Source: CAD feature listing. Evaluate the final solid. Frame: model axes, mm. A direction names the side the tool comes from. Give positions to 0.01 mm unless a question says otherwise; leave off trailing zeros. Loops run counter-clockwise (first coordinate to the right, second up) from the corner with the lowest first, then second, coordinate; pieces in that order, holes last.
```python
from build123d import *

# Parameters (mm, degrees)
RESSALTO_EXTRUS_O1_DEPTH = 3
ESBO_O2_W                = 40
ESBO_O2_H                = 3
ESBO_O2_W_2              = 3
ESBO_O2_H_2              = 40
CORTE_EXTRUS_O1_DEPTH    = 436.556992799
ESBO_O3_R                = 1.5
CORTE_EXTRUS_O2_DEPTH    = 436.556992799


with BuildPart() as part:
    # Esboço1 → Ressalto-extrusão1 (new body)
    with BuildSketch(Plane.XY):
        with BuildLine():
            Line((-241.20368795, -59.651351358), (-241.20368795, -29.651351358))
            ThreePointArc((-241.20368795, -29.651351358), (-246.107895674, -13.213553147), (-259.217101951, -2.150046733))
            ThreePointArc((-259.217101951, -2.150046733), (-264.561513741, -3.018769002), (-265.981323334, -8.243858139))
            ThreePointArc((-265.981323334, -8.243858139), (-265.003447457, -13.909864328), (-265.583076332, -19.630344878))
            ThreePointArc((-265.583076332, -19.630344878), (-271.11591561, -26.364097317), (-279.829636843, -26.200406546))
            ThreePointArc((-279.829636843, -26.200406546), (-306.442768457, 34.527322411), (-252.007526665, 72.381256019))
            ThreePointArc((-252.007526665, 72.381256019), (-244.422773084, 74.999120757), (-241.20368795, 82.348895826))
            Line((-241.20368795, 82.348895826), (-241.20368795, 98.348401458))
            ThreePointArc((-241.20368795, 98.348401458), (-237.984602816, 105.698176528), (-230.399849235, 108.316041265))
            ThreePointArc((-230.399849235, 108.316041265), (-175.964607443, 146.169974874), (-202.577739058, 206.897703831))
            ThreePointArc((-202.577739058, 206.897703831), (-211.29146029, 207.061394601), (-216.824299569, 200.327642163))
            ThreePointArc((-216.824299569, 200.327642163), (-217.403928444, 194.607161612), (-216.426052566, 188.941155423))
            ThreePointArc((-216.426052566, 188.941155423), (-217.845862159, 183.716066286), (-223.190273949, 182.847344017))
            ThreePointArc((-223.190273949, 182.847344017), (-236.299480227, 193.910850432), (-241.20368795, 210.348648642))
            Line((-241.20368795, 210.348648642), (-241.20368795, 240.348648642))
            Line((-241.20368795, 240.348648642), (-211.20368795, 240.348648642))
            ThreePointArc((-211.20368795, 240.348648642), (-194.76588974, 245.252856366), (-183.702383325, 258.362062643))
            ThreePointArc((-183.702383325, 258.362062643), (-184.571105594, 263.706474433), (-189.796194731, 265.126284027))
            ThreePointArc((-189.796194731, 265.126284027), (-195.46220092, 264.148408149), (-201.182681471, 264.728037024))
            ThreePointArc((-201.182681471, 264.728037024), (-207.916433909, 270.260876302), (-207.752743138, 278.974597535))
            ThreePointArc((-207.752743138, 278.974597535), (-147.025014182, 305.587729149), (-109.171080573, 251.152487357))
            ThreePointArc((-109.171080573, 251.152487357), (-106.553215836, 243.567733776), (-99.203440766, 240.348648642))
            Line((-99.203440766, 240.348648642), (-83.203935134, 240.348648642))
            ThreePointArc((-83.203935134, 240.348648642), (-75.854160064, 237.129563509), (-73.236295327, 229.544809927))
            ThreePointArc((-73.236295327, 229.544809927), (-35.382361719, 175.109568135), (25.345367238, 201.72269975))
            ThreePointArc((25.345367238, 201.72269975), (25.509058009, 210.436420982), (18.775305571, 215.969260261))
            ThreePointArc((18.775305571, 215.969260261), (13.05482502, 216.548889136), (7.388818831, 215.571013258))
            ThreePointArc((7.388818831, 215.571013258), (2.163729694, 216.990822851), (1.295007425, 222.335234642))
            ThreePointArc((1.295007425, 222.335234642), (12.358513839, 235.444440919), (28.79631205, 240.348648642))
            Line((28.79631205, 240.348648642), (58.79631205, 240.348648642))
            Line((58.79631205, 240.348648642), (58.79631205, 210.348648642))
            ThreePointArc((58.79631205, 210.348648642), (63.700519773, 193.910850432), (76.809726051, 182.847344017))
            ThreePointArc((76.809726051, 182.847344017), (82.154137841, 183.716066286), (83.573947435, 188.941155423))
            ThreePointArc((83.573947435, 188.941155423), (82.596071557, 194.607161612), (83.175700432, 200.327642163))
            ThreePointArc((83.175700432, 200.327642163), (88.70853971, 207.061394601), (97.422260943, 206.89770383))
            ThreePointArc((97.422260943, 206.89770383), (124.035392557, 146.169974874), (69.600150765, 108.316041265))
            ThreePointArc((69.600150765, 108.316041265), (62.015397184, 105.698176528), (58.79631205, 98.348401458))
            Line((58.79631205, 98.348401458), (58.79631205, 82.348895826))
            ThreePointArc((58.79631205, 82.348895826), (55.577226916, 74.999120757), (47.992473335, 72.381256019))
            ThreePointArc((47.992473335, 72.381256019), (-6.442768457, 34.527322411), (20.170363157, -26.200406546))
            ThreePointArc((20.170363157, -26.200406546), (28.88408439, -26.364097317), (34.416923668, -19.630344878))
            ThreePointArc((34.416923668, -19.630344878), (34.996552543, -13.909864328), (34.018676666, -8.243858139))
            ThreePointArc((34.018676666, -8.243858139), (35.438486259, -3.018769002), (40.782898049, -2.150046733))
            ThreePointArc((40.782898049, -2.150046733), (53.892104326, -13.213553147), (58.79631205, -29.651351358))
            Line((58.79631205, -29.651351358), (58.79631205, -59.651351358))
            Line((58.79631205, -59.651351358), (28.79631205, -59.651351358))
            ThreePointArc((28.79631205, -59.651351358), (12.358513839, -64.555559081), (1.295007425, -77.664765358))
            ThreePointArc((1.295007425, -77.664765358), (2.163729694, -83.009177149), (7.388818831, -84.428986742))
            ThreePointArc((7.388818831, -84.428986742), (13.05482502, -83.451110864), (18.775305571, -84.030739739))
            ThreePointArc((18.775305571, -84.030739739), (25.509058009, -89.563579018), (25.345367238, -98.27730025))
            ThreePointArc((25.345367238, -98.27730025), (-35.382361719, -124.890431865), (-73.236295327, -70.455190073))
            ThreePointArc((-73.236295327, -70.455190073), (-75.854160064, -62.870436491), (-83.203935134, -59.651351358))
            Line((-83.203935134, -59.651351358), (-99.203440766, -59.651351358))
            ThreePointArc((-99.203440766, -59.651351358), (-106.553215836, -56.432266224), (-109.171080573, -48.847512643))
            ThreePointArc((-109.171080573, -48.847512643), (-147.025014182, 5.587729149), (-207.752743138, -21.025402465))
            ThreePointArc((-207.752743138, -21.025402465), (-207.916433909, -29.739123698), (-201.182681471, -35.271962976))
            ThreePointArc((-201.182681471, -35.271962976), (-195.46220092, -35.851591851), (-189.796194731, -34.873715973))
            ThreePointArc((-189.796194731, -34.873715973), (-184.571105594, -36.293525567), (-183.702383325, -41.637937357))
            ThreePointArc((-183.702383325, -41.637937357), (-194.76588974, -54.747143634), (-211.20368795, -59.651351358))
            Line((-211.20368795, -59.651351358), (-241.20368795, -59.651351358))
        make_face()
    extrude(amount=RESSALTO_EXTRUS_O1_DEPTH)

    # Esboço2 → Corte-extrusão1 (cut, through all)
    with BuildSketch(Plane(origin=(0, 0, 0), x_dir=(-1, 0, 0), z_dir=(0, 0, -1))):
        with Locations((147.203935134, 240.348648642)):
            Rectangle(ESBO_O2_W, ESBO_O2_H)
        with Locations((-58.79631205, 146.348895826)):
            Rectangle(ESBO_O2_W_2, ESBO_O2_H_2)
        with Locations((35.20368795, -59.651351358)):
            Rectangle(ESBO_O2_W, ESBO_O2_H)
        with Locations((241.20368795, 34.348401458)):
            Rectangle(ESBO_O2_W_2, ESBO_O2_H_2)
    extrude(amount=-CORTE_EXTRUS_O1_DEPTH, mode=Mode.SUBTRACT)

    # Esboço3 → Corte-extrusão2 (cut, through all)
    with BuildSketch(Plane.XY.offset(3)):
        with Locations((-228.70368795, 46.348648642)):
            Circle(ESBO_O3_R)
        with Locations((-47.20368795, -47.151351358)):
            Circle(ESBO_O3_R)
        with Locations((46.29631205, 134.348648642)):
            Circle(ESBO_O3_R)
        with Locations((-135.20368795, 227.848648642)):
            Circle(ESBO_O3_R)
        with Locations((-47.20368795, -72.151351358)):
            Circle(ESBO_O3_R)
        with Locations((-253.70368795, 46.348648642)):
            Circle(ESBO_O3_R)
        with Locations((-135.20368795, 252.848648642)):
            Circle(ESBO_O3_R)
        with Locations((71.29631205, 134.348648642)):
            Circle(ESBO_O3_R)
    extrude(amount=-CORTE_EXTRUS_O2_DEPTH, mode=Mode.SUBTRACT)


solid = part.part
```
(1) First-contact query: pin 1 (1.5 mm diameter, centred on x = -224, z = 1.5, fed in from -Y); pin 2 (0.9 mm diameter, centred on x = -34.5, z = 2, fed in from -Y); pin 3 (1.5 mm diameter, centred on y = -14.5, z = 2, fed in from -X). Flat tips, straight axial feed; report the tip coordinate or a pass-through.
A:
pin 1: stops at y = -59.65
pin 2: stops at y = -125.25
pin 3: stops at x = -295.73
(2) Ray query, line 1 along X through (y, z) = (18, 1.8); line 2 along X through (y, z) = (198.5, 2); line 3 along Y through (x, z) = (1.5, 2.5). Return the intervals inside material, ascending.
A:
line 1: x = -308.35 to -242.7, -239.7 to -8.35
line 2: x = -238.76 to -217.18, -190.57 to -65.97, 23.56 to 61.24, 82.82 to 109.43
line 3: y = -121.66 to -82.08, -77.21 to -10.25, 50.94 to 178.34, 217.92 to 222.79
(3) Reachability of faces 1 (the cylindrical face through (-194.56, -54.61, 1.48)), 2 (the cylindrical face through (-195, 245.1, 1.5)), 3 (the cylindrical face through (12.6, -64.4, 1.5)), 4 (the cylindrical face through (63.568, 194.115, 1.479)) from +Z, -Z, +X, -X, +Y, -Y: full face, straight path, thin tool, end or side. Return the list, or none.
A:
face 1: +Z, -Z, -Y
face 2: +Z, -Z, -X
face 3: +Z, -Z, +X
face 4: +Z, -Z, +Y
(4) Section B-B, the plane y = 154.5. Return the cut outline in (x, z).
A:
outline: (-174.33, 0) - (57.3, 0) - (57.3, 3) - (-174.33, 3) - close; (60.3, 0) - (125.67, 0) - (125.67, 3) - (60.3, 3) - close
(5) Section C-C, the plane z = 2. Count the separate pieces of the cut face and the enclosed holes in it, then the cut area to 3 significant figures.
A:
separate pieces: 1
enclosed holes: 12
area: 89,500 mm2
(6) Mould query, pull axis X, two halves, no side actions, for faces 5 (the cylindrical face through (-36.348, 175.392, 1.479)), 6 (the flat face through (-88, 93, 0)), 7 (the cylindrical face through (-34.412, -125.154, 1.479)). Classes: pulls with the +X half, pulls with the -X half, needs draft (parallel to the pull), parting line crosses it, or undercut.
A:
face 5: undercut
face 6: needs draft
face 7: parting line crosses it
(7) Section A-A, the plane x = -29. Return the cut outline in (y, z), then the cut area to 3 significant figures.
A:
outline: (-126.27, 0) - (-61.15, 0) - (-61.15, 3) - (-126.27, 3) - close; (-58.15, 0) - (173.73, 0) - (173.73, 3) - (-58.15, 3) - close
area: 891 mm2
